Could you check a few things on this model? Use its own coordinates, in mm. Face numbers are marked on the shaded views. A direction names the side the tool comes from. Give positions to 0.01 mm unless a question says otherwise; leave off trailing zeros. Loops run counter-clockwise (first coordinate to the right, second up) from the corner with the lowest first, then second, coordinate; pieces in that order, holes last. Notation, with made-up numbers: M -38,4.25 L 19,4.25 A12 ccw 19,13.25 Z; hole C -2.5,88.5 d4. An arc over 180 degrees is marked long. Answer in a Markdown table with one row per item. Add a question column.
1. If we section it at D-D on x = 6: List the corners of the cut face in (y, z) for me.
2. If we section it at B-B on y = -20: Count the separate pieces of the cut face and the enclosed holes in it, then the cut area to 3 significant figures.
3. If we section it at C-C on x = 0: List the corners of the cut face in (y, z) for me, then the cut area to 3 significant figures.
4. If we section it at A-A on z = 0: List the corners of the cut face in (x, y) for me.
5. I need wall thicknesses on line 1 along X through (y, z) = (-33, 19); line 2 along Y through (x, z) = (-23.4, 0). Which ranges of each line are inside material? Lowest first, please. Write a range as from..to.
6. Which directions (+Z, -Z, +X, -X, +Y, -Y) give clear straight access to the entire face, cutting with the end or side of a thin tool? Please do the marked faces 4 and 5.
7. Thinking about a two-plate mould opening in Z: for the marked faces 1, 2 and 3, which applies, released by +Z, released by -Z, zero draft, split by the parting line, or undercut?
8. I'm going to push flat-ended pins straight in: pin 1 Ø9 at (x, y) = (0, -20) entering from -Z; pin 2 Ø10.5 at (y, z) = (-20, 0) entering from -X. Where does each tip first touch, or does it pass through?
```python
from build123d import *

# Parameters (mm, degrees)
SHS_C450_AS_50X50X2_3_SHS_C450_1_DEPTH = 150
SKETCH12_R                             = 3.25
CUT_EXTRUDE1_DEPTH                     = 10
SKETCH13_R                             = 3.25
CUT_EXTRUDE2_DEPTH                     = 10
SKETCH14_R                             = 7.5
CUT_EXTRUDE3_DEPTH                     = 10
SKETCH15_R                             = 7.5
CUT_EXTRUDE4_DEPTH                     = 10


with BuildPart() as part:
    # Sketch11 → Shs c450 as 50X50X2.3 SHS C450(1) (new body)
    with BuildSketch(Plane.ZX.offset(-75)):
        with BuildLine():
            Line((-20.4, -25), (20.4, -25))
            ThreePointArc((20.4, -25), (23.652691193, -23.652691193), (25, -20.4))
            Line((25, -20.4), (25, 20.4))
            ThreePointArc((25, 20.4), (23.652691193, 23.652691193), (20.4, 25))
            Line((20.4, 25), (-20.4, 25))
            ThreePointArc((-20.4, 25), (-23.652691193, 23.652691193), (-25, 20.4))
            Line((-25, 20.4), (-25, -20.4))
            ThreePointArc((-25, -20.4), (-23.652691193, -23.652691193), (-20.4, -25))
        make_face()
        with BuildLine():
            Line((-20.4, 22.7), (20.4, 22.7))
            ThreePointArc((20.4, 22.7), (22.026345597, 22.026345597), (22.7, 20.4))
            Line((22.7, 20.4), (22.7, -20.4))
            ThreePointArc((22.7, -20.4), (22.026345597, -22.026345597), (20.4, -22.7))
            Line((20.4, -22.7), (-20.4, -22.7))
            ThreePointArc((-20.4, -22.7), (-22.026345597, -22.026345597), (-22.7, -20.4))
            Line((-22.7, -20.4), (-22.7, 20.4))
            ThreePointArc((-22.7, 20.4), (-22.026345597, 22.026345597), (-20.4, 22.7))
        make_face(mode=Mode.SUBTRACT)
    extrude(amount=SHS_C450_AS_50X50X2_3_SHS_C450_1_DEPTH)

    # Sketch12 → Cut-Extrude1 (cut)
    with BuildSketch(Plane(origin=(25, 0, 0), x_dir=(0, 0, -1), z_dir=(1, 0, 0))):
        with Locations((0, -20)):
            Circle(SKETCH12_R)
    extrude(amount=-CUT_EXTRUDE1_DEPTH, mode=Mode.SUBTRACT)

    # Sketch13 → Cut-Extrude2 (cut)
    with BuildSketch(Plane(origin=(0, 0, -25), x_dir=(-1, 0, 0), z_dir=(0, 0, -1))):
        with Locations((0, -20)):
            Circle(SKETCH13_R)
    extrude(amount=-CUT_EXTRUDE2_DEPTH, mode=Mode.SUBTRACT)

    # Sketch14 → Cut-Extrude3 (cut)
    with BuildSketch(Plane.XY.offset(25)):
        with Locations((0, -20)):
            Circle(SKETCH14_R)
    extrude(amount=-CUT_EXTRUDE3_DEPTH, mode=Mode.SUBTRACT)

    # Sketch15 → Cut-Extrude4 (cut)
    with BuildSketch(Plane.ZY.offset(25)):
        with Locations((0, -20)):
            Circle(SKETCH15_R)
    extrude(amount=-CUT_EXTRUDE4_DEPTH, mode=Mode.SUBTRACT)


solid = part.part
```
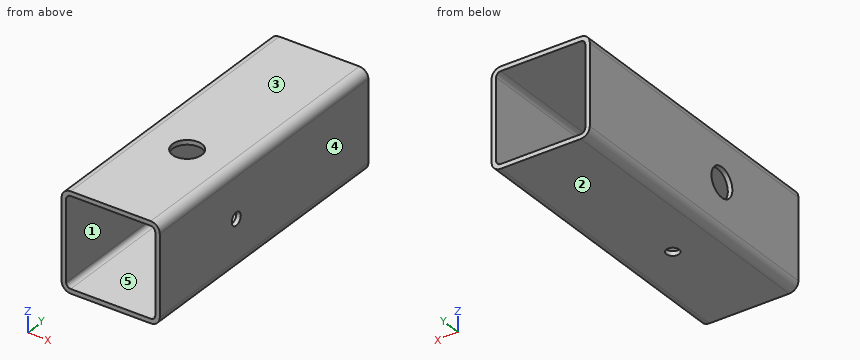
Results:
| question | item | result |
|---|---|---|
| 1 | outline | M -75,-25 L 75,-25 L 75,-22.7 L -75,-22.7 Z; M -75,22.7 L -24.5,22.7 L -24.5,25 L -75,25 Z; M -15.5,22.7 L 75,22.7 L 75,25 L -15.5,25 Z |
| 2 | separate pieces | 4 |
| 2 | enclosed holes | 0 |
| 2 | area | 326 mm2 |
| 3 | outline | M -75,-25 L -23.25,-25 L -23.25,-22.7 L -75,-22.7 Z; M -75,22.7 L -27.5,22.7 L -27.5,25 L -75,25 Z; M -16.75,-25 L 75,-25 L 75,-22.7 L -16.75,-22.7 Z; M -12.5,22.7 L 75,22.7 L 75,25 L -12.5,25 Z |
| 3 | area | 641 mm2 |
| 4 | outline | M -25,-75 L -22.7,-75 L -22.7,-27.5 L -25,-27.5 Z; M -25,-12.5 L -22.7,-12.5 L -22.7,75 L -25,75 Z; M 22.7,-75 L 25,-75 L 25,-23.25 L 22.7,-23.25 Z; M 22.7,-16.75 L 25,-16.75 L 25,75 L 22.7,75 Z |
| 5 | line 1 | -25..-22.7, 22.7..25 |
| 5 | line 2 | -75..-27.5, -12.5..75 |
| 6 | face 4 | +Z, -Z, +X, +Y, -Y |
| 6 | face 5 | +Y, -Y |
| 7 | face 1 | undercut |
| 7 | face 2 | released by -Z |
| 7 | face 3 | released by +Z |
| 8 | pin 1 | z = -25 |
| 8 | pin 2 | x = 22.7 |
